Verification items for this drawing (mm, ordinates from the low corner). A direction names the side the tool comes from. Coordinates: 2 decimals unless noted, no trailing zeros. Order: outer loops, then holes, each group sorted by start corner. A loop starts at its lowest first (then second) coordinate and runs counter-clockwise, first axis right, second up.
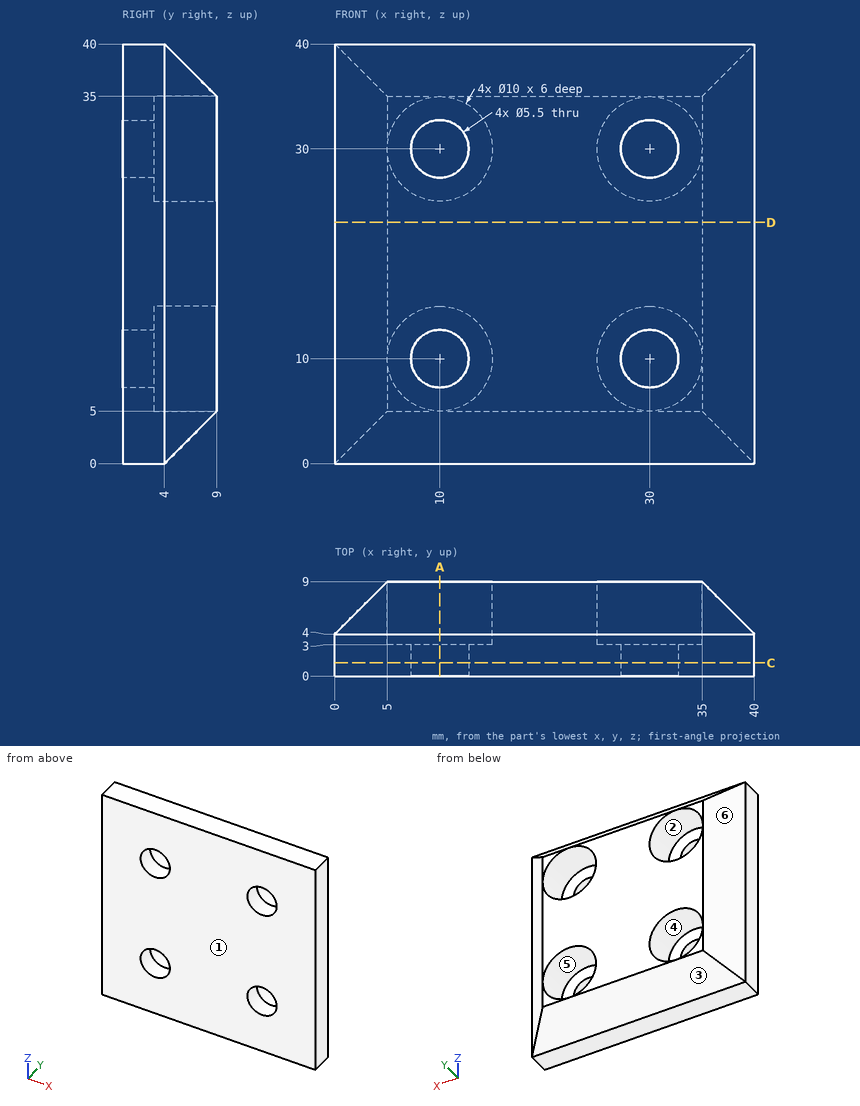
Item 1: Thickness scan on line 1 along X through (y, z) = (1.05, 30); line 2 along X through (y, z) = (8, 26.5); line 3 along Z through (x, y) = (9, 3.5). Record the ranges inside material, lowest first.
Item 2: Sectioned sample at C-C (y = 1.25). Record the cut outline in (x, z), and give its area (4 significant figures).
Item 3: Depth check by flat-ended pin: P1, Ø4, axis at y = 7, z = 26, coming from the +X side; P2, Ø8, axis at x = 10.5, z = 10, coming from the +Y side. Enter the tip coordinate at first touch or a pass-through.
Item 4: Sectioned sample at A-A (x = 10). Give the number of separate pieces and of enclosed holes in the cut face, and give its area (3 significant figures).
Item 5: Release check for a two-part mould opening along Z. For the marked faces 3, 4, 5 and 6 record: pulls with the +Z half, pulls with the -Z half, needs draft (parallel to the pull), parting line crosses it, or undercut.
Item 6: Sectioned sample at D-D (z = 23). Record the cut outline in (x, y).
Item 7: Tool access check on the marked faces 1 and 2. Record the directions out of +Z, -Z, +X, -X, +Y, -Y that give a thin tool (end or side, any length) a straight path to the whole face; none if there is none.
Geometry check:
1. line 1: x = 0 to 7.25, 12.75 to 27.25, 32.75 to 40
1. line 2: x = 4 to 6.43, 13.57 to 26.43, 33.57 to 36
1. line 3: z = 0 to 5.1, 14.9 to 25.1, 34.9 to 40
2. outline: (0, 0) - (40, 0) - (40, 40) - (0, 40) - close; hole circle Ø5.5 at (10, 10); hole circle Ø5.5 at (10, 30); hole circle Ø5.5 at (30, 10); hole circle Ø5.5 at (30, 30)
2. area: 1,505 mm2
3. P1: stops at x = 39
3. P2: stops at y = 3
4. separate pieces: 3
4. enclosed holes: 0
4. area: 182 mm2
5. face 3: pulls with the -Z half
5. face 4: undercut
5. face 5: undercut
5. face 6: needs draft
6. outline: (0, 0) - (40, 0) - (40, 4) - (35, 9) - (5, 9) - (0, 4) - close
7. face 1: +Z, -Z, +X, -X, -Y
7. face 2: +Y
